Job drawing, mm, ordinate dimensions from the low corner. One solid piece. Give positions to 0.01 mm unless a question says otherwise; leave off trailing zeros. Loops run counter-clockwise (first coordinate to the right, second up) from the corner with the lowest first, then second, coordinate; pieces in that order, holes last.
Item 1: Probe probe 1 along Z at (x, y) = (150.5, 5.75); probe 2 along Z at (x, y) = (132.5, 8); probe 3 along Z at (x, y) = (81.5, 17.25). List the from-to ranges inside material, lowest first.
Item 2: Saw through at C-C on z = 89. Give the cut face in (x, y).
Item 3: Saw through at B-B on y = 13.25. Give the cut face in (x, z).
Item 4: Saw through at A-A on x = 125. Give the cut face in (y, z).
Item 5: Mould opens along Z. For the marked faces 1, 2, 3 and 4 say: released by +Z, released by -Z, zero draft, split by the parting line, or undercut.
Item 6: Drop flat-ended pins along their axis: P1, Ø6.5, axis at y = 14.5, z = 33, coming from the -X side; P2, Ø6.5, axis at y = 14.5, z = 37.5, coming from the +X side; P3, Ø6, axis at x = 154.5, z = 211.5, coming from the +Y side. Give the stop position or say it passes through.
Item 7: Saw through at D-D on x = 29. Give the cut face in (y, z), plus the area to 3 significant figures.
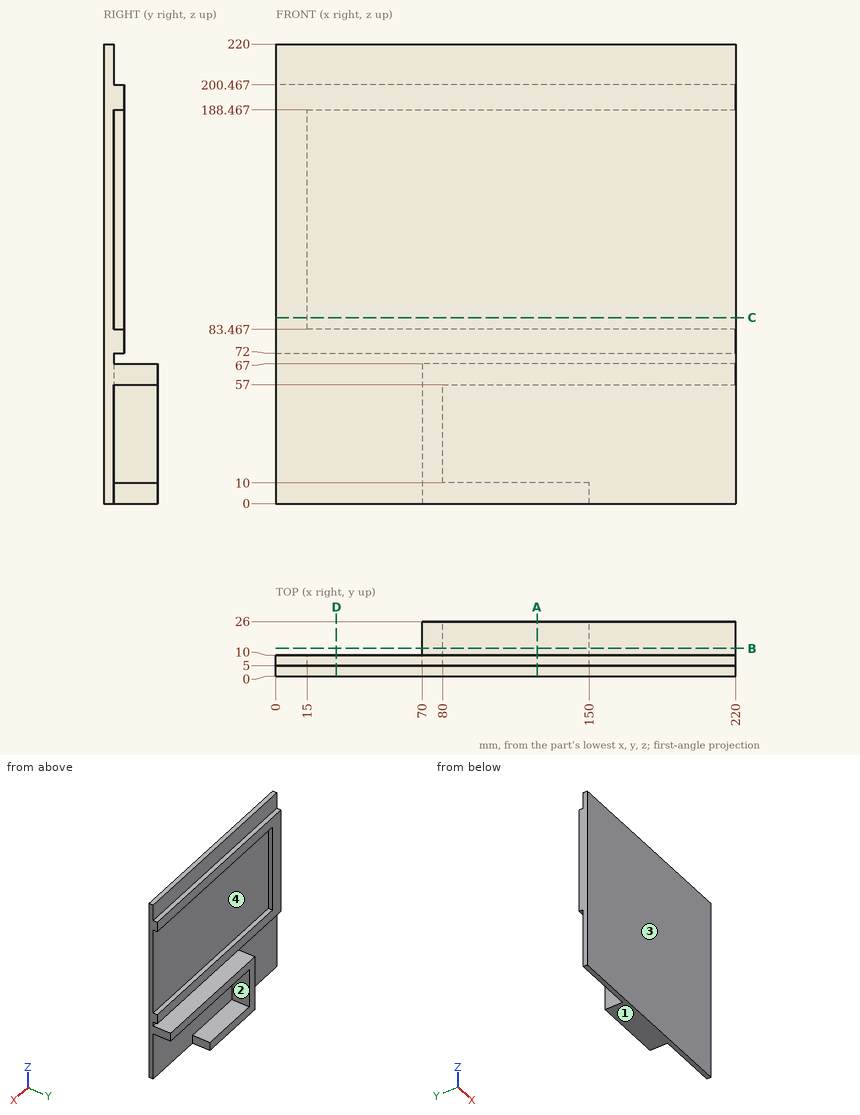
Results below:
1. probe 1: z = 57 to 67, 72 to 83.47, 188.47 to 200.47
1. probe 2: z = 0 to 10, 57 to 67, 72 to 83.47, 188.47 to 200.47
1. probe 3: z = 0 to 10, 57 to 67
2. outline: (0, 0) - (220, 0) - (220, 5) - (15, 5) - (15, 10) - (0, 10) - close
3. outline: (70, 0) - (150, 0) - (150, 10) - (80, 10) - (80, 57) - (220, 57) - (220, 67) - (70, 67) - close
4. outline: (0, 0) - (26, 0) - (26, 10) - (5, 10) - (5, 57) - (26, 57) - (26, 67) - (5, 67) - (5, 72) - (10, 72) - (10, 83.47) - (5, 83.47) - (5, 188.47) - (10, 188.47) - (10, 200.47) - (5, 200.47) - (5, 220) - (0, 220) - close
5. face 1: released by -Z
5. face 2: undercut
5. face 3: zero draft
5. face 4: undercut
6. P1: stops at x = 70
6. P2: stops at x = 80
6. P3: stops at y = 5
7. outline: (0, 0) - (5, 0) - (5, 72) - (10, 72) - (10, 83.47) - (5, 83.47) - (5, 188.47) - (10, 188.47) - (10, 200.47) - (5, 200.47) - (5, 220) - (0, 220) - close
7. area: 1,220 mm2
